Here's how the part is built. I have some questions about the finished solid (model axes, mm). Give positions to 0.01 mm unless a question says otherwise; leave off trailing zeros. Loops run counter-clockwise (first coordinate to the right, second up) from the corner with the lowest first, then second, coordinate; pieces in that order, holes last. Notation, with made-up numbers: (-31, 45.25) - (2, 45.25) arc R19 ccw to (2, 54.25) - close; hole circle Ø1 at (68.25, 64.25). An arc over 180 degrees is marked (long way). Return JSON: item names as keys, results as strings. Group by question number.
(1) If we section it at A-A (y = 133.35): Please give me the cut outline in (x, z), then the cut area to 3 significant figures.
(2) I need wall thicknesses on probe 1 along Y at (x, z) = (12, -50); probe 2 along Z at (x, y) = (29, 133); probe 3 along Z at (x, y) = (47.5, 124.5). Which ranges of each line are inside material? Lowest first, please. Write a range as [from, to].
(3) For P1, Ø4, axis at x = 20.5, y = 78.5, coming from the +Z side, with a flat end and sliding along its axis, tell me the tip position at first contact or that it passes through.
(4) If we section it at C-C (x = 25.5): Please give me the cut outline in (y, z).
(5) If we mould it in two halves opening along Y, with no side actions, what happens to faces 1 (the flat face through (50.8, 75, -50)), 2 (the cylindrical face through (25.756, 127.721, -64.377)), 3 (the flat face through (26, 0, -50)), 4 (the flat face through (26, 152.4, -50))? For each: released by +Y, released by -Y, zero draft, split by the parting line, or undercut.
(6) If we section it at B-B (z = -50.8): Please give me the cut outline in (x, y), then the cut area to 3 significant figures.
Autodesk Inventor part; units mm, degrees
ref_plane "YZ Plane" through (0, 0, 0) normal (1, 0, 0) x (0, 1, 0)
ref_plane "XZ Plane" through (0, 0, 0) normal (0, 1, 0) x (-1, 0, 0)
ref_plane "XY Plane" through (0, 0, 0) normal (0, 0, 1) x (1, 0, 0)
sketch "Sketch1" plane through (0, 0, 0) normal (0, 1, 0) x (-1, 0, 0)
  line L0 (0, 0) -> (-50.8, 0)
  line L1 (-50.8, 0) -> (-50.8, -101.6)
  line L2 (-50.8, -101.6) -> (0, -101.6)
  line L3 (0, -101.6) -> (0, 0)
  dimension "d0" = 50.8
  dimension "d1" = 101.6
extrude "Extrusion1" add sketch "Sketch1" along normal blind 152.4
sketch "Sketch2" plane through (50.8, 0, 0) normal (1, 0, 0) x (0, 0, -1)
  circle A0 centre (50.8, 133.35) radius 14.6973
  line L0 (101.6, 0) -> (101.6, 152.4)
  line L1 (0, 152.4) -> (101.6, 152.4)
  point P0 (0, 0)
  dimension "d4" = 50.8
  dimension "d5" = 19.05
extrude "Extrusion2" cut sketch "Sketch2" against normal up to next
properties part number "lifterBrace"
Values:
{
 "1": {"outline": "(0, -101.6) - (50.8, -101.6) - (50.8, -65.5) - (0, -65.5) - close; (0, -36.1) - (50.8, -36.1) - (50.8, 0) - (0, 0) - close", "area": "3,670 mm2"},
 "2": {"probe 1": "[0, 118.67], [148.03, 152.4]", "probe 2": "[-101.6, -65.49], [-36.11, 0]", "probe 3": "[-101.6, -62.53], [-39.07, 0]"},
 "3": {"P1": "z = 0"},
 "4": {"outline": "(0, -101.6) - (152.4, -101.6) - (152.4, 0) - (0, 0) - close; hole circle Ø29.39 at (133.35, -50.8)"},
 "5": {"face 1": "zero draft", "face 2": "undercut", "face 3": "released by -Y", "face 4": "released by +Y"},
 "6": {"outline": "(0, 0) - (50.8, 0) - (50.8, 118.65) - (0, 118.65) - close; (0, 148.05) - (50.8, 148.05) - (50.8, 152.4) - (0, 152.4) - close", "area": "6,250 mm2"}
}
